CAD build for the part. Positions are in the model's coordinates, mm. Coordinates: 2 decimals unless noted, no trailing zeros. Loops run counter-clockwise (first coordinate to the right, second up) from the corner with the lowest first, then second, coordinate; pieces in that order, holes last. Notation, with made-up numbers: (-14, 74) - (27, 74) arc R10 ccw to (27, 78) - close; hole circle Ø1 at (-30.5, -4.5). An arc over 180 degrees is marked (long way). Put each result on its own line as item: value.
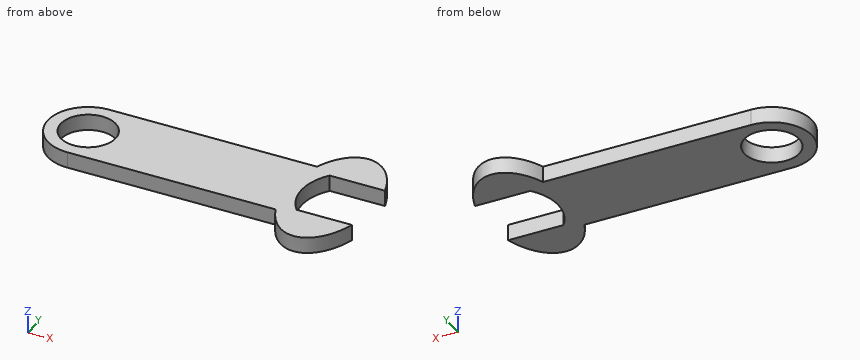
```python
from build123d import *

# Parameters (mm, degrees)
IZIM1_R                     = 17
Y_KSEKLIK_EKSTR_ZYON1_DEPTH = 10


with BuildPart() as part:
    # Çizim1 → Yükseklik-Ekstrüzyon1 (new body)
    with BuildSketch(Plane.XY):
        with BuildLine():
            Line((-50.538386463, 25), (78.943148636, 25))
            add(Edge.make_bspline(
                [(123.852580365, 20), (103.89283293, 89.629118064), (78.943148636, 25)],
                knots=[5.172942972, 5.172942972, 5.172942972, 7.264950664, 7.264950664, 7.264950664], degree=2, weights=[1, 0.501033423, 1]))
            Line((123.852580365, 20), (89.381621543, 20))
            ThreePointArc((89.381621543, 20), (82.361613537, 0), (89.381621543, -20))
            Line((89.381621543, -20), (123.852580365, -20))
            add(Edge.make_bspline(
                [(78.943148636, -25), (103.89283293, -89.629118064), (123.852580365, -20)],
                knots=[2.159827297, 2.159827297, 2.159827297, 4.251834989, 4.251834989, 4.251834989], degree=2, weights=[1, 0.501033423, 1]))
            Line((78.943148636, -25), (-50.538386463, -25))
            ThreePointArc((-50.538386463, -25), (-75.538386463, 0), (-50.538386463, 25))
        make_face()
        with Locations((-50.538386463, 0)):
            Circle(IZIM1_R, mode=Mode.SUBTRACT)
    extrude(amount=Y_KSEKLIK_EKSTR_ZYON1_DEPTH)


solid = part.part
```
Q1. Pin check, flat tips, straight feed: pin 1 Ø1 at (x, z) = (67.5, 6.5) entering from -Y; pin 2 Ø1 at (y, z) = (-20, 3) entering from -X; pin 3 Ø2 at (x, z) = (-6.5, 2) entering from +Y. Stop position of each tip, or through.
Determined:
pin 1: y = -25
pin 2: x = -66.18
pin 3: y = 25
Q2. Wall check: L1, parallel to X at y = -0.5, z = 5.75; L2, parallel to X at y = -6, z = 8; L3, parallel to Y at x = -12.5, z = 0.75. Give the ranges that are in metal, low to high. Write a range as from..to.
Determined:
L1: -75.53..-67.53, -33.55..82.37
L2: -74.81..-66.44, -34.63..82.93
L3: -25..25
Q3. Slice it at A-A, the plane y = 0. Give the cut face in (x, z).
Determined:
outline: (-75.54, 0) - (-67.54, 0) - (-67.54, 10) - (-75.54, 10) - close; (-33.54, 0) - (82.36, 0) - (82.36, 10) - (-33.54, 10) - close
Q4. Slice it at B-B, the plane x = 53. Give the cut face in (y, z).
Determined:
outline: (-25, 0) - (25, 0) - (25, 10) - (-25, 10) - close
